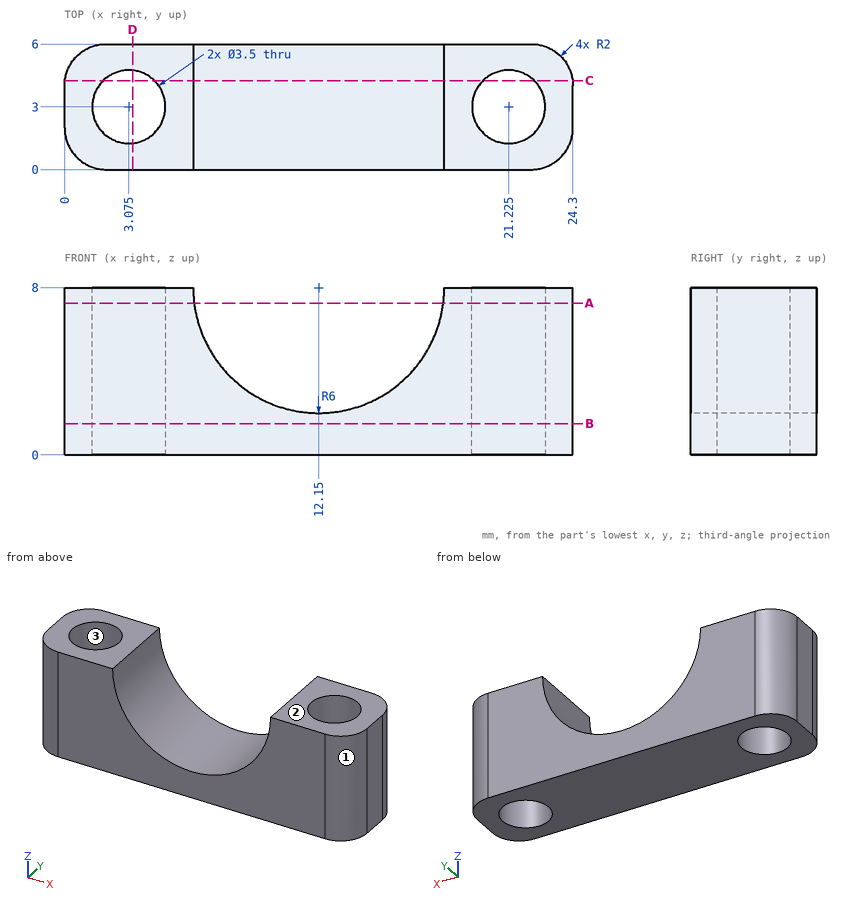
Answer from the drawing. Dimensions are ordinates in mm from the lowest x, y and z of the part. Round coordinates to 2 decimals unless told otherwise and drop trailing zeros. Write each loop counter-clockwise with the first axis right and the second up, starting at its lowest first coordinate (ties: lowest second). Pieces come first, ordered by that corner, then holes. Notation, with made-up numbers: (31, 27.5) -> (86, 27.5) arc R20 ccw to (86, 45.5) -> close; hole circle Ø3 at (71, 75.5). An arc over 180 degrees is marked (long way). Write each question's results on one line, items separated by ' | '.
1) The part is cut by section C-C (y = 4.25). Write down the section's boundary in (x, z), and give its area (3 significant figures).
Findings:
outline: (0.02, 0) -> (1.85, 0) -> (1.85, 8) -> (0.02, 8) -> close; (4.3, 0) -> (20, 0) -> (20, 8) -> (18.15, 8) arc R6 cw to (6.15, 8) -> (4.3, 8) -> close; (22.45, 0) -> (24.28, 0) -> (24.28, 8) -> (22.45, 8) -> close | area: 98.4 mm²
2) The part is cut by section D-D (x = 3.25). Write down the section's boundary in (y, z), and give its area (3 significant figures).
Findings:
outline: (0, 0) -> (1.26, 0) -> (1.26, 8) -> (0, 8) -> close; (4.74, 0) -> (6, 0) -> (6, 8) -> (4.74, 8) -> close | area: 20.1 mm²
3) For a pull along Y with two mould halves and no side action, classify the marked faces 1, 2 and 3 as +Y half, -Y half, draft (parallel to the pull), parting line (faces both ways), or undercut.
Findings:
face 1: -Y half | face 2: draft | face 3: undercut
4) Consider line 1 along X through (y, z) = (2, 6); line 2 along X through (y, z) = (1.5, 3.5); line 3 along Y through (x, z) = (3, 7.75). Determine where each line is inside the solid, lowest interval first. Write a range as [from, to].
Findings:
line 1: x = [0, 1.64], [4.51, 6.49], [17.81, 19.79], [22.66, 24.3] | line 2: x = [0.06, 2.17], [3.98, 8.18], [16.12, 20.32], [22.13, 24.24] | line 3: y = [0, 1.25], [4.75, 6]
5) The part is cut by section B-B (z = 1.5). Write down the section's boundary in (x, y) (3 decimals), and give its area (3 significant figures).
Findings:
outline: (0, 2) arc R2 ccw to (2, 0) -> (22.3, 0) arc R2 ccw to (24.3, 2) -> (24.3, 4) arc R2 ccw to (22.3, 6) -> (2, 6) arc R2 ccw to (0, 4) -> close; hole circle Ø3.5 at (3.075, 3); hole circle Ø3.5 at (21.225, 3) | area: 123 mm²
6) The part is cut by section A-A (z = 7.25). Write down the section's boundary in (x, y) (3 decimals).
Findings:
outline: (0, 2) arc R2 ccw to (2, 0) -> (6.197, 0) -> (6.197, 6) -> (2, 6) arc R2 ccw to (0, 4) -> close; (18.103, 0) -> (22.3, 0) arc R2 ccw to (24.3, 2) -> (24.3, 4) arc R2 ccw to (22.3, 6) -> (18.103, 6) -> close; hole circle Ø3.5 at (3.075, 3); hole circle Ø3.5 at (21.225, 3)
